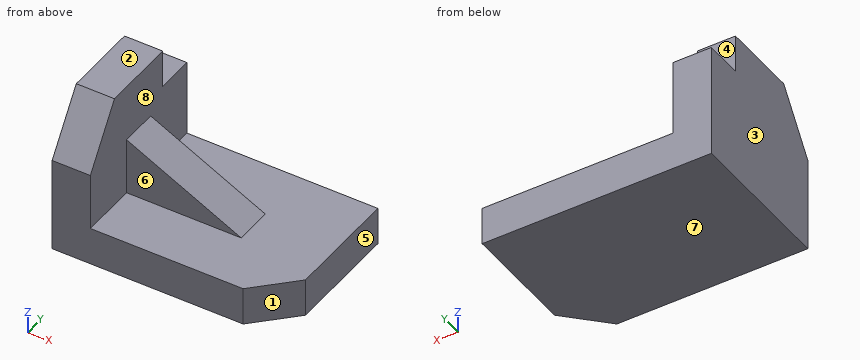
```python
from build123d import *

# Parameters (mm, degrees)
F0_W      = 60
F0_H      = 40
F1_DEPTH  = 40
F2_W      = 60
F2_H      = 40
F3_DEPTH  = 40.001
F5_DEPTH  = 10.001
F6_W      = 20
F6_H      = 20
F7_DEPTH  = 10.001
F9_DEPTH  = 10.001
F12_DEPTH = 10


with BuildPart() as f1:
    # F0 (on Front) → F1 (new body)
    with BuildSketch(Plane.XZ):
        with Locations((30, 20)):
            Rectangle(F0_W, F0_H)
    extrude(amount=-F1_DEPTH)

    # F2 (on face) → F3 (cut, through all)
    with BuildSketch(Plane.XZ):
        with Locations((40, 30)):
            Rectangle(F2_W, F2_H)
    extrude(amount=-F3_DEPTH, mode=Mode.SUBTRACT)

    # F4 (on face) → F5 (cut, through all)
    with BuildSketch(Plane.YZ.offset(10)):
        Polygon((-10, 25), (0, 25), (10, 40), (10, 50), (-10, 50), align=None)
    extrude(amount=-F5_DEPTH, mode=Mode.SUBTRACT)

    # F6 (on face) → F7 (cut, through all)
    with BuildSketch(Plane.YZ.offset(10)):
        with Locations((40, 40)):
            Rectangle(F6_W, F6_H)
    extrude(amount=-F7_DEPTH, mode=Mode.SUBTRACT)

    # F8 (on face) → F9 (cut, through all)
    with BuildSketch(Plane.XY.offset(10)):
        Polygon((60, 10), (50, 0), (50, -10), (70, -10), (70, 10), align=None)
    extrude(amount=-F9_DEPTH, mode=Mode.SUBTRACT)

    # F11 (on offset) → F12 (join)
    with BuildSketch(Plane.XZ.offset(-25)):
        Polygon((40, 10), (10, 25), (5, 25), (5, 5), (40, 5), align=None)
    extrude(amount=F12_DEPTH)


solid = f1.part
```
Here's how the part is built. I have some questions about the finished solid (model axes, mm). Face numbers are marked on the shaded views. A direction names the side the tool comes from. Round coordinates to 2 decimals unless told otherwise and drop trailing zeros. Write each loop counter-clockwise with the first axis right and the second up, starting at its lowest first coordinate (ties: lowest second). Pieces come first, ordered by that corner, then holes.
Q1. If we mould it in two halves opening along X, with no side actions, what happens to the marked faces 1, 2 and 3? For each: +X half, -X half, draft (parallel to the pull), parting line (faces both ways), or undercut.
Q2. If we section it at D-D on y = 20.5: Write out the boundary of the cut face in (x, z).
Q3. If we section it at A-A on z = 19: Write out the boundary of the cut face in (x, y).
Q4. Please list where these lines run through material, in increasing order: probe 1 along Z at (x, y) = (38, 7); probe 2 along Y at (x, z) = (26, 13.5).
Q5. Will these pins go through, and if not, where does the flat tip stop? P1, Ø10, axis at x = 19.5, y = 29.5, coming from the +Z side; P2, Ø10, axis at y = 24.5, z = 27, coming from the +X side; P3, Ø5, axis at x = 4, y = 37.5, coming from the +Z side.
Q6. Which directions (+Z, -Z, +X, -X, +Y, -Y) give clear straight access to the entire face, cutting with the end or side of a thin tool? Please do the marked faces 4, 5, 6, 7 and 8.
Q7. If we section it at B-B on x = 17: Write out the boundary of the cut face in (y, z).
Q8. If we section it at C-C on y = 35: Write out the boundary of the cut face in (x, z), plus the area to 3 significant figures.
Answer below:
1. face 1: +X half
1. face 2: draft
1. face 3: -X half
2. outline: (0, 0) - (60, 0) - (60, 10) - (40, 10) - (10, 25) - (10, 40) - (0, 40) - close
3. outline: (0, 0) - (10, 0) - (10, 15) - (22, 15) - (22, 25) - (10, 25) - (10, 40) - (0, 40) - close
4. probe 1: z = 0 to 10
4. probe 2: y = 15 to 25
5. P1: stops at z = 21.34
5. P2: stops at x = 16
5. P3: stops at z = 30
6. face 4: +Z, +X, -X, +Y
6. face 5: +Z, -Z, +X, +Y, -Y
6. face 6: +Z, +X, -Y
6. face 7: -Z, +X, -X, +Y, -Y
6. face 8: +Z, +X
7. outline: (0, 0) - (40, 0) - (40, 10) - (25, 10) - (25, 21.5) - (15, 21.5) - (15, 10) - (0, 10) - close
8. outline: (0, 0) - (60, 0) - (60, 10) - (10, 10) - (10, 30) - (0, 30) - close
8. area: 800 mm2
